Autodesk Inventor part; units mm, degrees
ref_plane "YZ Plane" through (0, 0, 0) normal (1, 0, 0) x (0, 1, 0)
ref_plane "XZ Plane" through (0, 0, 0) normal (0, 1, 0) x (-1, 0, 0)
ref_plane "XY Plane" through (0, 0, 0) normal (0, 0, 1) x (1, 0, 0)
sketch "Sketch1" plane through (0, 0, 0) normal (0, 0, 1) x (1, 0, 0)
  line L0 (-13.5, 42) -> (13.5, 42) construction
  line L1 (13.5, 42) -> (13.5, -42) construction
  line L2 (13.5, -42) -> (-13.5, -42) construction
  line L3 (-13.5, -42) -> (-13.5, 42) construction
  line L4 (-10, 30) -> (10, 30)
  line L5 (10, 30) -> (10, -30)
  line L6 (10, -30) -> (-10, -30)
  line L7 (-10, -30) -> (-10, 30)
  circle A0 centre (-8, 37) radius 2.025
  circle A1 centre (8, 37) radius 2.025
  circle A2 centre (8, -37) radius 2.025
  circle A3 centre (-8, -37) radius 2.025
  line L8 (-16.5, 45) -> (16.5, 45)
  line L9 (16.5, 45) -> (16.5, -45)
  line L10 (16.5, -45) -> (-16.5, -45)
  line L11 (-16.5, -45) -> (-16.5, 45)
  line L12 (-23.1, 0) -> (23.1, 0)
  point P0 (0, 0)
  dimension "d0" = 27
  dimension "d8" = 4.05
  dimension "d9" = 5
  dimension "d10" = 5.5
  dimension "d11" = 4.05
  dimension "d12" = 5.5
  dimension "d13" = 4.05
  dimension "d14" = 5
  dimension "d15" = 4.05
  dimension "d17" = 33
  dimension "d19" = 16.5
  dimension "d29" = 5.5
  dimension "d31" = 5
  dimension "d66" = 15
  dimension "d68" = 8
  dimension "d69" = 8
  dimension "d71" = 60
  dimension "d72" = 15
  dimension "d73" = 8
  dimension "d76" = 30
  dimension "d77" = 20
  dimension "d79" = 8
extrude "Extrusion1" add sketch "Sketch1" along normal blind 12 contours A0 | A1 | A2 | A3
extrude "Extrusion2" add sketch "Sketch1" against normal blind 4 contours L7 L12 L11 L8 L9 L5 L4 | L4 L5 L12 L7 | L12 L5 L6 L7 | L7 L6 L5 L12 L9 L10 L11 | A0 | A1 | A2 | A3
extrude "Extrusion3" [suppressed]
sketch "Sketch2" plane through (0, 0, 12) normal (0, 0, 1) x (1, 0, 0)
  line L0 (-10, -30) -> (10, -30)
  line L1 (10, -30) -> (10, 30)
  line L2 (10, 30) -> (-10, 30)
  line L3 (-10, 30) -> (-10, -30)
  circle A0 centre (-8, 37) radius 2.025
  circle A1 centre (8, 37) radius 2.025
  circle A2 centre (8, -37) radius 2.025
  circle A3 centre (-8, -37) radius 2.025
  point P0 (0, 0)
extrude "Extrusion4" [suppressed]
sketch "Sketch3" plane through (0, 0, -4) normal (0, 0, -1) x (-1, 0, 0)
  line L0 (31.5, 60) -> (-31.5, 60)
  line L1 (-31.5, 60) -> (-31.5, -60)
  line L2 (-31.5, -60) -> (31.5, -60)
  line L3 (31.5, -60) -> (31.5, 60)
  line L4 (16.5, -45) -> (16.5, 45)
  line L5 (-16.5, 45) -> (-16.5, -45)
  line L6 (-16.5, -45) -> (16.5, -45)
  line L7 (16.5, 45) -> (-16.5, 45)
  point P0 (0, 0)
  dimension "d32" = 15
  dimension "d33" = 15
  dimension "d34" = 15
  dimension "d35" = 15
extrude "Extrusion5" [suppressed]
sketch "Sketch4" plane through (-31.5, -38, 0) normal (0, 0, 1) x (1, 0, 0)
  line L0 (0, 0) -> (0, 76)
  line L1 (0, 76) -> (63, 76)
  line L2 (0, 0) -> (63, 0)
  line L3 (63, 0) -> (63, 76)
  line L4 (63, 76) -> (0, 76)
  line L5 (0, 76) -> (0, 0)
  line L6 (60.5, 73.5) -> (2.5, 73.5)
  line L7 (2.5, 73.5) -> (2.5, 2.5)
  line L8 (2.5, 2.5) -> (60.5, 2.5)
  line L9 (60.5, 2.5) -> (60.5, 73.5)
  point P0 (31.5, 38)
  dimension "d38" = 2.5
  dimension "d39" = 2.5
  dimension "d40" = 2.5
  dimension "d41" = 2.5
extrude "Extrusion6" [suppressed]
sketch "Sketch6" plane through (0, 0, -4) normal (0, 0, -1) x (-1, 0, 0)
  line L0 (-10, 30) -> (-10, -30)
  line L1 (10, -30) -> (-10, -30)
  line L2 (-10, 30) -> (10, 30)
  line L3 (10, 30) -> (10, -30)
  line L4 (10, -30) -> (-10, -30)
  line L5 (-10, -30) -> (-10, 30)
  point P0 (0, 0)
extrude "Extrusion7" add sketch "Sketch6" against normal blind 14
sketch "Sketch7" plane through (0, 0, -4) normal (0, 0, -1) x (-1, 0, 0)
  circle A0 centre (8, -37) radius 2.025
  circle A1 centre (8, -37) radius 2.1
  circle A2 centre (-8, -37) radius 2.025
  circle A3 centre (-8, -37) radius 2.1
  circle A4 centre (-8, 37) radius 2.025
  circle A5 centre (-8, 37) radius 2.1
  circle A6 centre (8, 37) radius 2.025
  circle A7 centre (8, 37) radius 2.1
  point P0 (0, 0)
  dimension "d58" = 4.2
  dimension "d59" = 4.2
  dimension "d60" = 4.2
  dimension "d61" = 4.2
extrude "Extrusion8" [suppressed]
fillet "Fillet1" [suppressed]
fillet "Fillet2" [suppressed]
fillet "Fillet3" radius 2 8 edges at (-10.025, -37, 12) (5.975, -37, 12) (5.975, 37, 12) (-10.025, 37, 12) (5.975, -37, 0) (-10.025, -37, 0) (5.975, 37, 0) (-10.025, 37, 0)
sketch "Sketch8" plane through (0, 0, 0) normal (0, 0, 1) x (1, 0, 0)
  point P0 (0, 0)
properties part number "Long PDMS Chamber-Mold"
Input: part model. Units: mm. Frame: model coordinates. A direction names the side the tool comes from. Round coordinates to 2 decimals unless told otherwise and drop trailing zeros. Loops run counter-clockwise (first coordinate to the right, second up) from the corner with the lowest first, then second, coordinate; pieces in that order, holes last.
1) Section query C-C on y = -25.5. Return the cut outline in (x, z), plus the area to 3 significant figures.
Ans:
outline: (-16.5, -4) - (16.5, -4) - (16.5, 0) - (10, 0) - (10, 10) - (-10, 10) - (-10, 0) - (-16.5, 0) - close
area: 332 mm2
2) Pull-direction query (Y, two-part tool) for faces 4 (the flat face through (0, 45, -2)), 5 (the flat face through (0, -45, -2)), 6 (the flat face through (0, 1, -4)), 7 (the flat face through (0, 0, 10)); classes: released by +Y, released by -Y, zero draft, split by the parting line, or undercut.
Ans:
face 4: released by +Y
face 5: released by -Y
face 6: zero draft
face 7: undercut
3) Section query B-B on x = -1.5. Return the cut outline in (y, z), plus the area to 3 significant figures.
Ans:
outline: (-45, -4) - (45, -4) - (45, 0) - (30, 0) - (30, 10) - (-30, 10) - (-30, 0) - (-45, 0) - close
area: 960 mm2
4) Pin query (flat end, axial travel): pin 1 (3 mm diameter, centred on x = 9.5, y = 11, fed in from +Z); pin 2 (3 mm diameter, centred on y = 15, z = 5.5, fed in from -X); pin 3 (1 mm diameter, centred on y = -4.5, z = 5.5, fed in from +X); pin 4 (1.5 mm diameter, centred on y = -26.5, z = 0.5, fed in from +X). Return the tip coordinate at first contact, or that it passes through.
Ans:
pin 1: stops at z = 10
pin 2: stops at x = -10
pin 3: stops at x = 10
pin 4: stops at x = 16.5
5) Set-up query: faces 1 (the flat face through (11, 11, 0)), 2 (the flat face through (-10, 0, 5)), 3 (the flat face through (10, 0, 5)). Return all of +Z, -Z, +X, -X, +Y, -Y with unobstructed straight access to the full face (end or side cutting, diameter ignored); none if empty.
Ans:
face 1: +Z
face 2: +Z, -X
face 3: +Z, +X
6) Section query A-A on z = 8.25. Return the cut outline in (x, y) (3 decimals).
Ans:
outline: circle Ø4.05 at (-8, -37); circle Ø4.05 at (-8, 37); (-10, -30) - (10, -30) - (10, 30) - (-10, 30) - close; circle Ø4.05 at (8, -37); circle Ø4.05 at (8, 37)
7) Material intervals for line 1 (Y direction, x = 8, z = 7.5) (3 decimals); line 2 (Y direction, x = -1, z = 7); line 3 (Z direction, x = -10.5, y = 12), sorted ascending.
Ans:
line 1: y = -39.025 to -34.975, -30 to 30, 34.975 to 39.025
line 2: y = -30 to 30
line 3: z = -4 to 0
